Can you work these out from the model? Positions are in its coordinate system, mm. Coordinates: 2 decimals unless noted, no trailing zeros. Write each loop counter-clockwise with the first axis right and the second up, starting at its lowest first coordinate (ties: lowest second). Pieces come first, ordered by that corner, then holes. Notation, with made-up numbers: M 46,-33.75 L 105,-33.75 A24 ccw 105,-9.75 Z; hole C 65.5,30.25 d5. An arc over 180 degrees is marked long. Answer as a JSON object with one key per item and string values. Group by question number.
from build123d import *


with BuildPart() as part:
    # Sketch1 → Revolve1 (revolve)
    with BuildSketch(Plane.XY, mode=Mode.PRIVATE) as revolve1_sk:
        with BuildLine():
            Line((12.7, 22.86), (12.7, 44.45))
            Line((12.7, 44.45), (-12.7, 44.45))
            Line((-12.7, 44.45), (-12.7, 22.86))
            ThreePointArc((-12.7, 22.86), (-7.62, 17.78), (-12.7, 12.7))
            Line((-12.7, 12.7), (-12.7, 6.35))
            Line((-12.7, 6.35), (12.7, 6.35))
            Line((12.7, 6.35), (12.7, 12.7))
            ThreePointArc((12.7, 12.7), (7.62, 17.78), (12.7, 22.86))
        make_face()
    revolve(revolve1_sk.sketch.rotate(Axis((12.7, 0, 0), (-1, 0, 0)), 90), axis=Axis((12.7, 0, 0), (-1, 0, 0)))


solid = part.part
Q1. Will these pins go through, and if not, where does the flat tip stop? pin 1 (3 mm diameter, centred on x = -5.5, y = 33, fed in from +Z); pin 2 (10 mm diameter, centred on x = -8.5, z = -19.5, fed in from +Y); pin 3 (6 mm diameter, centred on x = 5, y = 9.5, fed in from +Z); pin 4 (20.5 mm diameter, centred on y = 0, z = 0, fed in from +X).
Q2. We'd pull the mould along Y, two halves only. Please class faces 1 (the flat face through (12.7, -6, 3)), 2 (the cylindrical face through (0.18, 3.86, 5.04)), 3 (the cylindrical face through (-0.2, -30, 32.8)): pulls with the +Y half, pulls with the -Y half, needs draft (parallel to the pull), parting line crosses it, or undercut.
Q3. Please list where these lines run through material, in increasing order: L1, parallel to Y at x = -6, z = 0; L2, parallel to Y at x = -10.25, z = -0.5; L3, parallel to Z at x = 7.25, y = -1.5.
Q4. If we section it at A-A on y = 0: List the corners of the cut face in (x, z) for me.
Q5. If we section it at C-C on x = -2.5: List the corners of the cut face in (y, z) for me, and give its area (3 significant figures).
Q6. If we section it at D-D on z = 37.5: List the corners of the cut face in (x, y) for me, and give its area (3 significant figures).
Reply:
{
 "1": {"pin 1": "z = 31.36", "pin 2": "y = 42.02", "pin 3": "z = 43.97", "pin 4": "x = 12.7"},
 "2": {"face 1": "needs draft", "face 2": "undercut", "face 3": "parting line crosses it"},
 "3": {"L1": "-44.45 to -6.35, 6.35 to 44.45", "L2": "-44.45 to -22.22, -13.32 to -6.33, 6.33 to 13.32, 22.22 to 44.45", "L3": "-44.42 to -6.17, 6.17 to 44.42"},
 "4": {"outline": "M -12.7,-44.45 L 12.7,-44.45 L 12.7,-22.86 A5.08 cw 12.7,-12.7 L 12.7,-6.35 L -12.7,-6.35 L -12.7,-12.7 A5.08 cw -12.7,-22.86 Z; M -12.7,6.35 L 12.7,6.35 L 12.7,12.7 A5.08 cw 12.7,22.86 L 12.7,44.45 L -12.7,44.45 L -12.7,22.86 A5.08 cw -12.7,12.7 Z"},
 "5": {"outline": "C 0,0 d88.9; hole C 0,0 d12.7", "area": "6,080 mm^2"},
 "6": {"outline": "M -12.7,-23.87 L 12.7,-23.87 L 12.7,23.87 L -12.7,23.87 Z", "area": "1,210 mm^2"}
}
